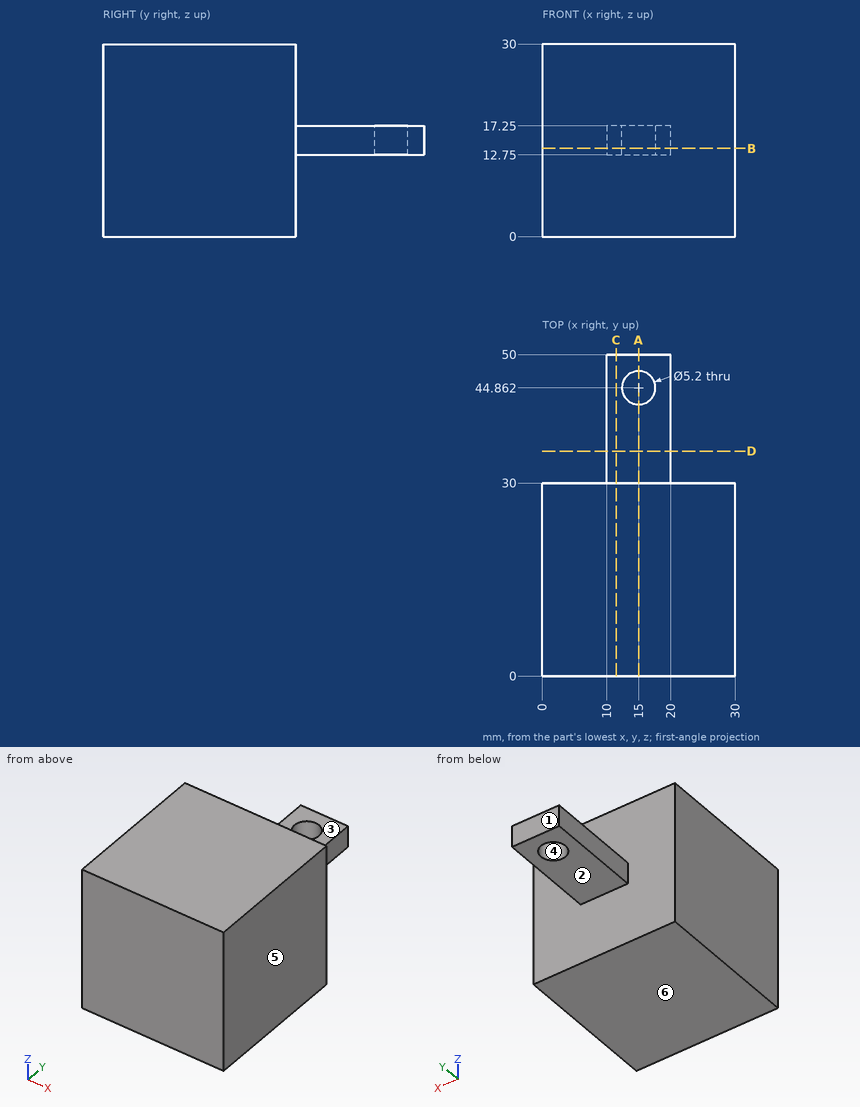
Source: three-view drawing plus pictorial views. Frame: mm from the lowest corner of the part. A direction names the side the tool comes from. Give positions to 0.01 mm unless a question says otherwise; leave off trailing zeros. Write each loop counter-clockwise with the first axis right and the second up, starting at its lowest first coordinate (ties: lowest second). Pieces come first, ordered by that corner, then holes. Notation, with made-up numbers: (-24.5, 69) -> (21.5, 69) arc R28 cw to (21.5, 98) -> close; hole circle Ø1 at (-11.75, -2). An arc over 180 degrees is marked (long way). Answer in a Markdown table with one row per item.
(1) Pin query (flat end, axial travel): pin 1 (5 mm diameter, centred on y = 37, z = 16, fed in from -X); pin 2 (3 mm diameter, centred on x = 12.5, y = 43.5, fed in from -Z); pin 3 (6 mm diameter, centred on x = 23, z = 26.5, fed in from +Y). Return the tip coordinate at first contact, or that it passes through.
Answers below:
| item | result |
|---|---|
| pin 1 | x = 10 |
| pin 2 | z = 12.75 |
| pin 3 | y = 30 |
(2) Section query C-C on x = 11.5. Return loops of the section in (y, z).
Answers below:
| item | result |
|---|---|
| outline | (0, 0) -> (30, 0) -> (30, 12.75) -> (50, 12.75) -> (50, 17.25) -> (30, 17.25) -> (30, 30) -> (0, 30) -> close |
(3) Section query A-A on x = 15. Return loops of the section in (y, z).
Answers below:
| item | result |
|---|---|
| outline | (0, 0) -> (30, 0) -> (30, 12.75) -> (42.26, 12.75) -> (42.26, 17.25) -> (30, 17.25) -> (30, 30) -> (0, 30) -> close; (47.46, 12.75) -> (50, 12.75) -> (50, 17.25) -> (47.46, 17.25) -> close |
(4) Ray query, line 1 along Y through (x, z) = (15, 15.85); line 2 along Y through (x, z) = (15.5, 25); line 3 along X through (y, z) = (44.5, 13) (1 decimal). Return the intervals inside material, ascending. Write a range as [from, to].
Answers below:
| item | result |
|---|---|
| line 1 | [0, 42.26], [47.46, 50] |
| line 2 | [0, 30] |
| line 3 | [10, 12.4], [17.6, 20] |
(5) Set-up query: the marked faces 1, 2 and 3. Return all of +Z, -Z, +X, -X, +Y, -Y with unobstructed straight access to the full face (end or side cutting, diameter ignored); none if empty.
Answers below:
| item | result |
|---|---|
| face 1 | +Z, -Z, +X, -X, +Y |
| face 2 | -Z, +X, -X, +Y |
| face 3 | +Z, +X, -X, +Y |
(6) Section query D-D on y = 35. Return loops of the section in (x, z), then the cut area to 3 significant figures.
Answers below:
| item | result |
|---|---|
| outline | (10, 12.75) -> (20, 12.75) -> (20, 17.25) -> (10, 17.25) -> close |
| area | 45.0 mm^2 |
(7) Draft query along X for the marked faces 4, 5 and 6. Return one class per face: +X half, -X half, draft (parallel to the pull), parting line (faces both ways), or undercut.
Answers below:
| item | result |
|---|---|
| face 4 | undercut |
| face 5 | +X half |
| face 6 | draft |
(8) Section query B-B on z = 13.75. Return loops of the section in (x, y).
Answers below:
| item | result |
|---|---|
| outline | (0, 0) -> (30, 0) -> (30, 30) -> (20, 30) -> (20, 50) -> (10, 50) -> (10, 30) -> (0, 30) -> close; hole circle Ø5.2 at (15, 44.86) |
